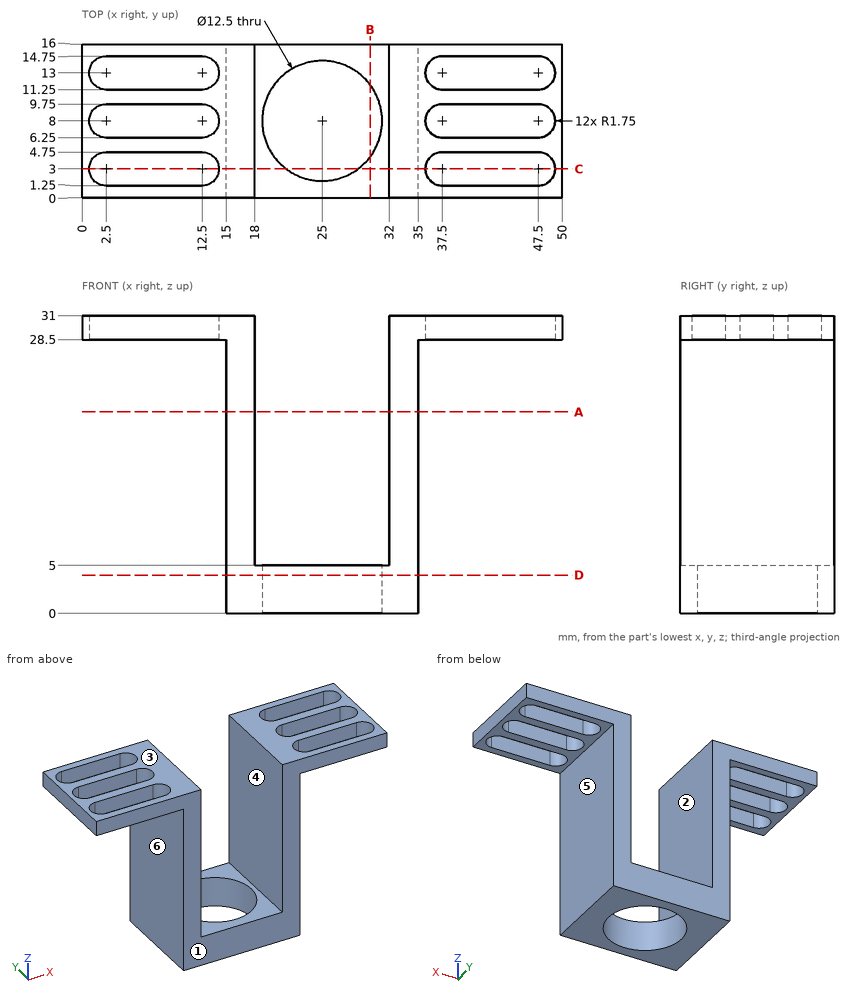
Verification items for this drawing (mm, ordinates from the low corner). A direction names the side the tool comes from. Coordinates: 2 decimals unless noted, no trailing zeros. Order: outer loops, then holes, each group sorted by start corner. A loop starts at its lowest first (then second) coordinate and runs counter-clockwise, first axis right, second up. Notation, with made-up numbers: M 86,51.5 L 143,51.5 A32 ccw 143,89.5 Z; hole C -30,32 d2. An arc over 180 degrees is marked long. Use CSV: the item, a comma, the result in double quotes.
Item 1: Cross-section at C-C on y = 3. Record the cut outline in (x, z).
Returned:
outline,"M 0,28.5 L 0.75,28.5 L 0.75,31 L 0,31 Z; M 14.25,28.5 L 15,28.5 L 15,0 L 21.25,0 L 21.25,5 L 18,5 L 18,31 L 14.25,31 Z; M 28.75,0 L 35,0 L 35,28.5 L 35.75,28.5 L 35.75,31 L 32,31 L 32,5 L 28.75,5 Z; M 49.25,28.5 L 50,28.5 L 50,31 L 49.25,31 Z"
Item 2: Gauge pin test, flat ends, axial feed: pin 1 Ø5 at (y, z) = (8.5, 11) entering from -X; pin 2 Ø10 at (x, z) = (41, 23) entering from +Y; pin 3 Ø4.5 at (x, y) = (42.5, 10) entering from -Z. Record the tip position at first contact, or that the pin passes through.
Returned:
pin 1,"stops at x = 15"
pin 2,"passes through"
pin 3,"stops at z = 28.5"
Item 3: Cross-section at A-A on z = 21. Record the cut outline in (x, y), then the cut area to 3 significant figures.
Returned:
outline,"M 15,0 L 18,0 L 18,16 L 15,16 Z; M 32,0 L 35,0 L 35,16 L 32,16 Z"
area,"96.0 mm2"
Item 4: Cross-section at B-B on x = 30. Record the cut outline in (y, z).
Returned:
outline,"M 0,0 L 4.25,0 L 4.25,5 L 0,5 Z; M 11.75,0 L 16,0 L 16,5 L 11.75,5 Z"
Item 5: Mould release check, pull along X, two halves, no side actions. Record for the marked faces 3, 4, 5 and 6: pulls with the +X half, pulls with the -X half, needs draft (parallel to the pull), parting line crosses it, or undercut.
Returned:
face 3,"needs draft"
face 4,"undercut"
face 5,"pulls with the +X half"
face 6,"pulls with the -X half"
Item 6: Thickness scan on line 1 along X through (y, z) = (5.5, 19); line 2 along Y through (x, z) = (25, 1.05); line 3 along Y through (x, z) = (5.5, 30.5). Record the ranges inside material, lowest first.
Returned:
line 1,"x = 15 to 18, 32 to 35"
line 2,"y = 0 to 1.75, 14.25 to 16"
line 3,"y = 0 to 1.25, 4.75 to 6.25, 9.75 to 11.25, 14.75 to 16"
Item 7: Tool access check on the marked faces 1 and 2. Record the directions out of +Z, -Z, +X, -X, +Y, -Y that give a thin tool (end or side, any length) a straight path to the whole face; none if there is none.
Returned:
face 1,"+Z, -Z, +X, -X, -Y"
face 2,"+Z, +Y, -Y"
Item 8: Cross-section at D-D on z = 4. Record the cut outline in (x, y).
Returned:
outline,"M 15,0 L 35,0 L 35,16 L 15,16 Z; hole C 25,8 d12.5"
